Design review of the part built by this model. Coordinates are the model's own, in mm. A direction names the side the tool comes from. Coordinates: 2 decimals unless noted, no trailing zeros. Write each loop counter-clockwise with the first axis right and the second up, starting at its lowest first coordinate (ties: lowest second). Pieces come first, ordered by that corner, then holes.
Q1. Take a section at A-A (y = 47). Give the boundary of the cut face in (x, z).
Q2. Take a section at C-C (y = 31.5). Give the boundary of the cut face in (x, z).
Q3. Take a section at D-D (x = 108.5). Give the boundary of the cut face in (y, z).
Q4. Take a section at B-B (z = -102.5). Give the boundary of the cut face in (x, y).
Q5. Insertion check: pin 1 (6 mm diameter, centred on y = 76.5, z = -130.5, fed in from +X); pin 2 (22 mm diameter, centred on x = 12, y = 77.5, fed in from +Z); pin 3 (2 mm diameter, centred on x = 114.5, z = -20, fed in from +Y). Each pin has a flat end and moves straight along its axis. Give the tip position at first contact, or say it passes through.
Q6. Mouldability with a two-part tool opening along Z and no side actions: class faces 4 (the flat face through (131, 75, -148.5)), 5 (the flat face through (75, 35, -97.9)), 6 (the flat face through (50, 35, -52)), 7 (the flat face through (0, 32, -74)) as pulls with the +Z half, pulls with the -Z half, needs draft (parallel to the pull), parting line crosses it, or undercut.
Q7. For probe 1 along X at (y, z) = (34.5, -17); probe 2 along X at (y, z) = (71.5, -134); probe 3 along X at (y, z) = (39, -131.5), list the stretches that pass through material, from the lowest coordinate up.
Q8. Machinability: for faces 1 (the flat face through (1.5, 75, -131)), 2 (the flat face through (122, 35, -5)), 3 (the flat face through (150, 32, -74)), which of the approach directions +Z, -Z, +X, -X, +Y, -Y give a long, thin tool a straight path to every point of the face, cutting with its end or side? Answer none if there is none.
```python
from build123d import *

# Parameters (mm, degrees)
SKETCH1_W                       = 150
SKETCH1_H                       = 150
BOSS_EXTRUDE1_DEPTH             = 65
SHELL1_T                        = -5
FILLET1_R                       = 2
BOSS_EXTRUDE2_DEPTH             = 20
CUT_EXTRUDE1_REACH              = 230.528
SKETCH3_W                       = 44
SKETCH3_H                       = 35
BOSS_EXTRUDE3_DEPTH             = 60
BOSS_EXTRUDE4_REACH             = 190.016
BOSS_EXTRUDE4_DIRECTION_2_REACH = 190.016


with BuildPart() as part:
    # Sketch1 → Boss-Extrude1 (new body)
    with BuildSketch(Plane(origin=(0, 0, 0), x_dir=(1, 0, 0), z_dir=(0, 1, 0))):
        with Locations((75, 75)):
            Rectangle(SKETCH1_W, SKETCH1_H)
    extrude(amount=BOSS_EXTRUDE1_DEPTH)

    # Shell1
    shell1_openings = [part.faces().sort_by_distance(p)[0] for p in [
        (75, 65, -75),
    ]]
    offset(amount=SHELL1_T, openings=shell1_openings, kind=Kind.INTERSECTION)

    # Fillet1
    fillet1_edges = [part.edges().sort_by_distance(p)[0] for p in [
        (0, 32.5, -150),
        (150, 32.5, -150),
        (150, 32.5, 0),
        (0, 32.5, 0),
    ]]
    fillet(fillet1_edges, radius=FILLET1_R)

    # Sketch2 → Boss-Extrude2 (add)
    with BuildSketch(Plane(origin=(0, 65, 0), x_dir=(1, 0, 0), z_dir=(0, 1, 0))):
        Polygon((1.5, 113.5), (1.5, 148.5), (36.5, 148.5), (36.5, 146.5), (3.5, 146.5), (3.5, 113.5), align=None)
        Polygon((148.5, 113.5), (148.5, 148.5), (113.5, 148.5), (113.5, 146.5), (146.5, 146.5), (146.5, 113.5), align=None)
        Polygon((148.5, 36.5), (148.5, 1.5), (113.5, 1.5), (113.5, 3.5), (146.5, 3.5), (146.5, 36.5), align=None)
        Polygon((1.5, 36.5), (1.5, 1.5), (36.5, 1.5), (36.5, 3.5), (3.5, 3.5), (3.5, 36.5), align=None)
    extrude(amount=BOSS_EXTRUDE2_DEPTH)

    # Sketch3 → Cut-Extrude1 (cut, up to next)
    with BuildSketch(Plane.XY, mode=Mode.PRIVATE) as cut_extrude1_sk1:
        with Locations((75, 22.5)):
            Rectangle(SKETCH3_W, SKETCH3_H)
    cut_extrude1_tool1 = extrude(cut_extrude1_sk1.sketch, amount=-CUT_EXTRUDE1_REACH, mode=Mode.PRIVATE) & part.part
    add(cut_extrude1_tool1.solids().sort_by_distance((75, 22.5, 0))[0], mode=Mode.SUBTRACT)

    # Sketch4 → Boss-Extrude3 (add)
    with BuildSketch(Plane(origin=(0, 5, 0), x_dir=(1, 0, 0), z_dir=(0, 1, 0))):
        Polygon((53, 5), (53, 94.9), (97, 94.9), (97, 5), (100, 5), (100, 97.9), (50, 97.9), (50, 5), align=None)
    extrude(amount=BOSS_EXTRUDE3_DEPTH)

    # Sketch7 → Boss-Extrude4 (add, up to next)
    with BuildSketch(Plane(origin=(75, 0, 0), x_dir=(0, 0, -1), z_dir=(1, 0, 0)), mode=Mode.PRIVATE) as boss_extrude4_sk1:
        Polygon((94.9, 42.158643577), (0, 5), (94.9, 5), align=None)
    boss_extrude4_tool1 = extrude(boss_extrude4_sk1.sketch, amount=BOSS_EXTRUDE4_REACH, mode=Mode.PRIVATE) - part.part
    add(boss_extrude4_tool1.solids().sort_by_distance((75, 17.386215, -63.266667))[0])

    # Sketch7 → Boss-Extrude4 direction 2 (add, up to next)
    with BuildSketch(Plane(origin=(75, 0, 0), x_dir=(0, 0, -1), z_dir=(1, 0, 0)), mode=Mode.PRIVATE) as boss_extrude4_direction_2_sk1:
        Polygon((94.9, 42.158643577), (0, 5), (94.9, 5), align=None)
    boss_extrude4_direction_2_tool1 = extrude(boss_extrude4_direction_2_sk1.sketch, amount=-BOSS_EXTRUDE4_DIRECTION_2_REACH, mode=Mode.PRIVATE) - part.part
    add(boss_extrude4_direction_2_tool1.solids().sort_by_distance((75, 17.386215, -63.266667))[0])


solid = part.part
```
Response:
1. outline: (0, -148) arc R2 ccw to (2, -150) - (148, -150) arc R2 ccw to (150, -148) - (150, -2) arc R2 ccw to (148, 0) - (2, 0) arc R2 ccw to (0, -2) - close; hole (5, -145) - (145, -145) - (145, -5) - (100, -5) - (100, -97.9) - (50, -97.9) - (50, -5) - (5, -5) - close; hole (53, -94.9) - (97, -94.9) - (97, -5) - (53, -5) - close
2. outline: (0, -148) arc R2 ccw to (2, -150) - (148, -150) arc R2 ccw to (150, -148) - (150, -2) arc R2 ccw to (148, 0) - (97, 0) - (97, -67.68) - (53, -67.68) - (53, 0) - (2, 0) arc R2 ccw to (0, -2) - close; hole (5, -145) - (145, -145) - (145, -5) - (100, -5) - (100, -97.9) - (50, -97.9) - (50, -5) - (5, -5) - close
3. outline: (0, -150) - (65, -150) - (65, -145) - (5, -145) - (5, -5) - (65, -5) - (65, 0) - (0, 0) - close
4. outline: (0, 0) - (150, 0) - (150, 65) - (145, 65) - (145, 5) - (5, 5) - (5, 65) - (0, 65) - close
5. pin 1: stops at x = 148.5
5. pin 2: stops at z = -1.5
5. pin 3: stops at y = 5
6. face 4: pulls with the -Z half
6. face 5: undercut
6. face 6: undercut
6. face 7: needs draft
7. probe 1: x = 0 to 5, 50 to 53, 97 to 100, 145 to 150
7. probe 2: x = 1.5 to 3.5, 146.5 to 148.5
7. probe 3: x = 0 to 5, 145 to 150
8. face 1: +Z, -Z, -X, +Y
8. face 2: +Y
8. face 3: +Z, -Z, +X, +Y, -Y
